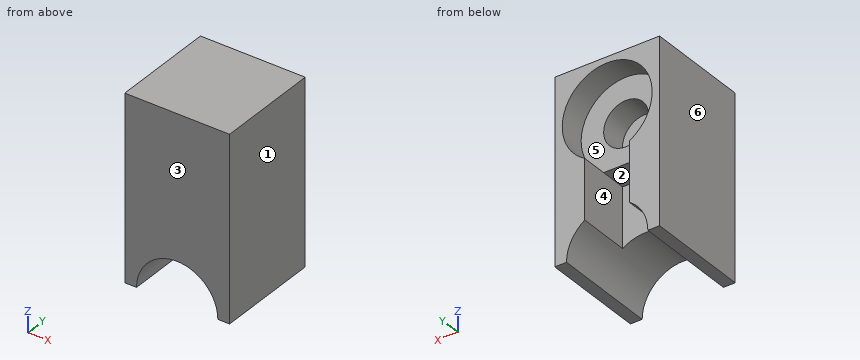
Autodesk Inventor part; units mm, degrees
ref_plane "YZ Plane" through (0, 0, 0) normal (1, 0, 0) x (0, 1, 0)
ref_plane "XZ Plane" through (0, 0, 0) normal (0, 1, 0) x (-1, 0, 0)
ref_plane "XY Plane" through (0, 0, 0) normal (0, 0, 1) x (1, 0, 0)
sketch "Sketch1" plane through (0, 0, 0) normal (0, 1, 0) x (-1, 0, 0)
  line L0 (5.2933, 33.6678) -> (56.0933, 33.6678)
  line L1 (56.0933, 33.6678) -> (56.0933, -55.2322)
  line L2 (56.0933, -55.2322) -> (5.2933, -55.2322)
  line L3 (5.2933, -55.2322) -> (5.2933, 33.6678)
  point P0 (0, 0)
  dimension "d0" = 50.8
  dimension "d1" = 88.9
extrude "Extrusion1" add sketch "Sketch1" along normal blind 50.8
sketch "Sketch2" plane through (0, 50.8, 0) normal (0, 1, 0) x (1, 0, 0)
  circle A0 centre (-30.6933, -8.9925) radius 21.7895
  circle A1 centre (-30.6933, -8.9925) radius 10.8785
  line L0 (-5.2933, 55.2322) -> (-56.0933, 55.2322)
  line L1 (-19.8148, 9.8871) -> (-41.5719, 9.8871)
  line L2 (-41.5719, 9.8871) -> (-41.5719, 55.2322)
  line L3 (-41.5719, 55.2322) -> (-19.8148, 55.2322)
  line L4 (-19.8148, 55.2322) -> (-19.8148, 9.8871)
  circle A2 centre (-30.6933, 55.2322) radius 19.7044
  point P0 (0, 0)
extrude "Extrusion2" cut sketch "Sketch2" against normal up to next contours A2 L2 L0 L4 | L4 L0 A2 | A2 L0 L2 | L0 A2
extrude "Extrusion3" cut sketch "Sketch2" against normal blind 12.7 contours A0 L1 | L1 A0
extrude "Extrusion4" cut sketch "Sketch2" against normal blind 25.4 contours A1
extrude "Extrusion5" cut sketch "Sketch2" against normal blind 25.4 contours L1 A0 | A0 L2 A2 L4 | A2 L2 L0 L4 picked at (-29.9354, 10.8174)
properties part number "7.2 part 2"
For this review, take the finished solid that the model builds, in its own axes (mm). Face numbers are marked on the shaded views. A direction names the side the tool comes from. Give positions to 0.01 mm unless a question says otherwise; leave off trailing zeros. Order: outer loops, then holes, each group sorted by start corner. A loop starts at its lowest first (then second) coordinate and runs counter-clockwise, first axis right, second up.
1) Take a section at A-A (y = 39.5). Give the boundary of the cut face in (x, z).
2) Take a section at C-C (x = -10). Give the boundary of the cut face in (y, z), then the cut area to 3 significant figures.
3) The part is to be moulded in two halves that separate along X. For the marked faces 1, 2 and 3, say which applies: released by +X, released by -X, zero draft, split by the parting line, or undercut.
4) Wall thickness on line 1 (X direction, y = 31, z = -12.5); line 2 (Y direction, x = -23.5, z = 14.5); line 3 (X direction, y = 26, z = 6): over which ranges is each line inside the solid? List them lowest first.
5) For the marked faces 4, 5 and 6, list the 3-axis set-ups (+Z, -Z, +X, -X, +Y, -Y) from which the entire face can be reached by the end or side of a thin tool; tool diameter is ignored.
6) Take a section at B-B (z = -42.5). Give the boundary of the cut face in (x, y), then the cut area to 3 significant figures.
7) Take a section at D-D (y = 32.5). Give the boundary of the cut face in (x, z).
8) Insertion check: pin 1 (5 mm diameter, centred on x = -12.5, z = -18, fed in from -Y); pin 2 (4 mm diameter, centred on x = -26.5, y = 33.5, fed in from -Z); pin 3 (17.5 mm diameter, centred on x = -34.5, z = 8.5, fed in from +Y); pin 4 (2 mm diameter, centred on x = -40, z = 9, fed in from +Y). Each pin has a flat end and moves straight along its axis. Give the tip position at first contact, or say it passes through.
Derived:
1. outline: (-56.09, -55.23) - (-50.4, -55.23) arc R19.7 cw to (-41.57, -38.8) - (-41.57, -9.89) arc R21.79 cw (long way) to (-19.81, -9.89) - (-19.81, -38.8) arc R19.7 cw to (-10.99, -55.23) - (-5.29, -55.23) - (-5.29, 33.67) - (-56.09, 33.67) - close
2. outline: (0, -55.23) - (50.8, -55.23) - (50.8, 2.17) - (38.1, 2.17) - (38.1, 15.82) - (50.8, 15.82) - (50.8, 33.67) - (0, 33.67) - close
2. area: 4,340 mm2
3. face 1: released by +X
3. face 2: undercut
3. face 3: zero draft
4. line 1: x = -56.09 to -41.57, -19.81 to -5.29
4. line 2: y = 0 to 25.4
4. line 3: x = -56.09 to -41.15, -20.23 to -5.29
5. face 4: -Z, +Y
5. face 5: +Y
5. face 6: +Z, -Z, -X, +Y, -Y
6. outline: (-56.09, 0) - (-45.73, 0) - (-45.73, 50.8) - (-56.09, 50.8) - close; (-15.65, 0) - (-5.29, 0) - (-5.29, 50.8) - (-15.65, 50.8) - close
6. area: 1,050 mm2
7. outline: (-56.09, -55.23) - (-50.4, -55.23) arc R19.7 cw to (-41.57, -38.8) - (-41.57, -9.89) - (-19.81, -9.89) - (-19.81, -38.8) arc R19.7 cw to (-10.99, -55.23) - (-5.29, -55.23) - (-5.29, 33.67) - (-56.09, 33.67) - close; hole circle Ø21.76 at (-30.69, 8.99)
8. pin 1: stops at y = 0
8. pin 2: stops at z = -9.89
8. pin 3: stops at y = 38.1
8. pin 4: stops at y = 25.4
